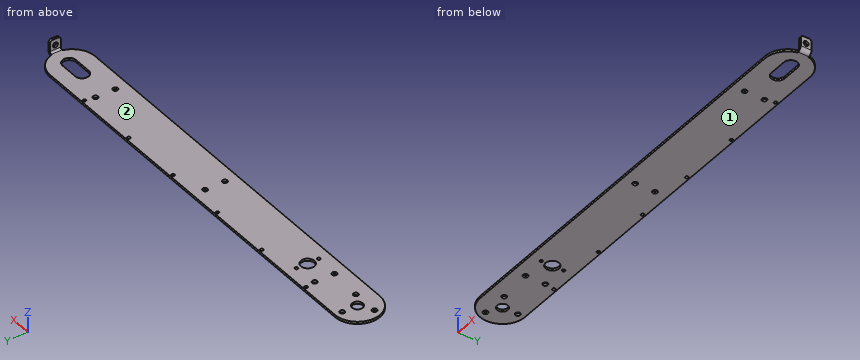
```python
from build123d import *
from build123d.topology import SkipClean

# Parameters (mm, degrees)
AUFSATZ_LINEAR_AUSTRAGEN1_DEPTH        = 2.5
SKIZZE7_W                              = 2.5
SKIZZE7_H                              = 6
AUFSATZ_LINEAR_AUSTRAGEN2_DEPTH        = 14
VERRUNDUNG2_R                          = 3
F_5_5_5_5_DURCHMESSER_BOHRUNG1_D       = 5.5
KREISMUSTER1_COUNT                     = 3
DURCHGANGSLOCH_F_R_M51_D               = 5.5
DURCHGANGSLOCH_F_R_M51_DEPTH           = 9.5
DURCHGANGSLOCH_F_R_M51_TIP             = 1.652366702
F_3_5_3_5_DURCHMESSER_BOHRUNG1_D       = 3.5
DURCHGANGSLOCH_F_R_M52_D               = 5.5
SPIEGELN2_AT_THE_SECOND_PLANE_COPY_1_D = 5.5
SCHNITT_LINEAR_AUSTRAGEN1_REACH        = 482.355
SKIZZE19_R                             = 7.5
VOLUMENK_RPER_START                    = -6
VOLUMENK_RPER_UMWANDELN1_DEPTH         = 12
VOLUMENK_RPER_UMWANDELN1_2_DEPTH       = 12


# Read off the part's stored shape, not the designer's step: Volumenkörper umwandeln1
with BuildPart() as part:
    # Skizze1 → Aufsatz-Linear austragen1 (new body)
    with BuildSketch(Plane.XY):
        with BuildLine():
            Line((-6, 0), (-25, 0))
            ThreePointArc((-25, 0), (-17.67766953, 17.67766953), (0, 25))
            Line((0, 25), (450, 25))
            ThreePointArc((450, 25), (465.411035007, 19.685019685), (474.269322199, 6))
            Line((474.269322199, 6), (479.5, 6))
            Line((479.5, 6), (479.5, 0))
            Line((479.5, 0), (477, 0))
            Line((477, 0), (475, 0))
            Line((475, 0), (462.5, 0))
            ThreePointArc((462.5, 0), (460.303300859, 5.303300859), (455, 7.5))
            Line((455, 7.5), (450, 7.5))
            Line((450, 7.5), (435, 7.5))
            ThreePointArc((435, 7.5), (429.696699141, 5.303300859), (427.5, 0))
            Line((427.5, 0), (6, 0))
            ThreePointArc((6, 0), (0, 6), (-6, 0))
        make_face()
    extrude(amount=-AUFSATZ_LINEAR_AUSTRAGEN1_DEPTH)

    # Skizze7 → Aufsatz-Linear austragen2 (add)
    with BuildSketch(Plane.XY):
        with Locations((478.25, 3)):
            Rectangle(SKIZZE7_W, SKIZZE7_H)
    extrude(amount=AUFSATZ_LINEAR_AUSTRAGEN2_DEPTH)

    # Verrundung2
    verrundung2_edges = [part.edges().sort_by_distance(p)[0] for p in [
        (478.25, 6, 14),
    ]]
    fillet(verrundung2_edges, radius=VERRUNDUNG2_R)

    # Spiegeln1: part across plane


with BuildPart() as part_1:
    with SkipClean():  # the faces are left unmerged after this step: merging them gives an invalid solid
        add(part.part)
        add(part.part.mirror(Plane(origin=(6, 0, -2.5), x_dir=(0, 0, 1), z_dir=(0, -1, 0))))

    # Ø5.5 (5.5) Durchmesser Bohrung1 (through all)
    with Locations(Plane.XY):
        with Locations((0, 17)):
            f_5_5_5_5_durchmesser_bohrung1 = Hole(F_5_5_5_5_DURCHMESSER_BOHRUNG1_D / 2)

    # Kreismuster1: Ø5.5 (5.5) Durchmesser Bohrung1 ×3 about axis
    with SkipClean():  # the faces are left unmerged after this step: merging them gives an invalid solid
        kreismuster1_axis = Axis((0, 0, 0), (0, 0, 1))
        for i in range(1, KREISMUSTER1_COUNT):
            add(f_5_5_5_5_durchmesser_bohrung1.rotate(kreismuster1_axis, i * 360 / KREISMUSTER1_COUNT), mode=Mode.SUBTRACT)

    # Durchgangsloch für M51
    with Locations(Plane(origin=(479.5, 0, 0), x_dir=(0, 0, -1), z_dir=(1, 0, 0))):
        with Locations((-7, 0)):
            Hole(DURCHGANGSLOCH_F_R_M51_D / 2, depth=DURCHGANGSLOCH_F_R_M51_DEPTH)
            with Locations((0, 0, -(DURCHGANGSLOCH_F_R_M51_DEPTH + DURCHGANGSLOCH_F_R_M51_TIP / 2))):  # 118° drill point
                Cone(0, DURCHGANGSLOCH_F_R_M51_D / 2, DURCHGANGSLOCH_F_R_M51_TIP, mode=Mode.SUBTRACT)

    # Ø3.5 (3.5) Durchmesser Bohrung1 (through all)
    with Locations(Plane.XY):
        with Locations((400, 22), (330, 22), (260, 22), (190, 22), (120, 22), (50, 22)):
            Hole(F_3_5_3_5_DURCHMESSER_BOHRUNG1_D / 2)

    # Durchgangsloch für M52 (through all)
    with Locations(Plane.XY):
        with Locations((52, 11), (225, 11)):
            durchgangsloch_f_r_m52 = Hole(DURCHGANGSLOCH_F_R_M52_D / 2)

    # Spiegeln2: Durchgangsloch für M52 across plane
    with SkipClean():  # the faces are left unmerged after this step: merging them gives an invalid solid
        add(durchgangsloch_f_r_m52.mirror(Plane(origin=(225, 0, 0), x_dir=(0, 0, 1), z_dir=(1, 0, 0))), mode=Mode.SUBTRACT)

    # Spiegeln2 at the second plane: Durchgangsloch für M52 across plane
    with SkipClean():  # the faces are left unmerged after this step: merging them gives an invalid solid
        add(durchgangsloch_f_r_m52.mirror(Plane.ZX), mode=Mode.SUBTRACT)

    # Spiegeln2 at the second plane copy 1 (through all)
    with Locations(Plane(origin=(450, 0, 0), x_dir=(-1, 0, 0), z_dir=(0, 0, 1))):
        with Locations((52, 11), (225, 11)):
            Hole(SPIEGELN2_AT_THE_SECOND_PLANE_COPY_1_D / 2)

    # Skizze19 → Schnitt-Linear austragen1 (cut, up to next)
    with BuildSketch(Plane.XY, mode=Mode.PRIVATE) as schnitt_linear_austragen1_sk1:
        with Locations((78.75, 0)):
            Circle(SKIZZE19_R)
    schnitt_linear_austragen1_tool1 = extrude(schnitt_linear_austragen1_sk1.sketch, amount=-SCHNITT_LINEAR_AUSTRAGEN1_REACH, mode=Mode.PRIVATE) & part_1.part
    add(schnitt_linear_austragen1_tool1.solids().sort_by_distance((78.75, 0, 0))[0], mode=Mode.SUBTRACT)

    # Skizze22 → Durchgangsloch für M31 (revolve, cut)
    with SkipClean():  # the faces are left unmerged after this step: merging them gives an invalid solid
        with BuildSketch(Plane(origin=(78.75, 12.5, 0), x_dir=(0, -1, 0), z_dir=(1, 0, 0))):
            Polygon((0, 0), (0, 3.771463052), (1.7, 2.75), (1.7, 0), align=None)
        durchgangsloch_f_r_m31 = revolve(axis=Axis((78.75, 12.5, 6.35), (0, 0, -1)), mode=Mode.SUBTRACT)

    # Spiegeln3: Durchgangsloch für M31 across plane
    with SkipClean():  # the faces are left unmerged after this step: merging them gives an invalid solid
        add(durchgangsloch_f_r_m31.mirror(Plane.ZX), mode=Mode.SUBTRACT)

    # Volumenkörper umwandeln1 outline → Volumenkörper umwandeln1 (cut)
    with SkipClean():  # the faces are left unmerged after this step: merging them gives an invalid solid
        with BuildSketch(Plane(origin=(0, 0, 0), x_dir=(1, 0, 0), z_dir=(0, 1, 0)).offset(VOLUMENK_RPER_START)):
            with BuildLine():
                Line((479.5, 2.5), (475, 2.5))
                ThreePointArc((475, 2.5), (478.181980515, 1.181980515), (479.5, -2))
                Line((479.5, -2), (479.5, 2.5))
            make_face()
        extrude(amount=VOLUMENK_RPER_UMWANDELN1_DEPTH, mode=Mode.SUBTRACT)

    # Volumenk_rper umwandeln1 2 outline → Volumenk_rper umwandeln1 2 (add)
    with BuildSketch(Plane(origin=(0, 0, 0), x_dir=(1, 0, 0), z_dir=(0, 1, 0)).offset(VOLUMENK_RPER_START)):
        with BuildLine():
            Line((477, 0), (475, 0))
            ThreePointArc((475, 0), (476.414213562, -0.585786438), (477, -2))
            Line((477, -2), (477, 0))
        make_face()
    extrude(amount=VOLUMENK_RPER_UMWANDELN1_2_DEPTH)


solid = part_1.part
```
The listing builds one solid part. Answer for the finished solid, in the listing's coordinates (mm). Face numbers are marked on the shaded views. A direction names the side the tool comes from. Coordinates: 2 decimals unless noted, no trailing zeros. Write each loop counter-clockwise with the first axis right and the second up, starting at its lowest first coordinate (ties: lowest second). Pieces come first, ordered by that corner, then holes.
Q1. Which of the six approach directions +Z, -Z, +X, -X, +Y, -Y give full straight-line access (tool end or side, diameter ignored) to the marked faces 1 and 2?
Returned:
face 1: -Z, +X, -X, +Y, -Y
face 2: +Z, -X, +Y, -Y
Q2. Find the intervals of material crossed by line 1 along Y through (x, z) = (78.75, -0.6); line 2 along Y through (x, z) = (477.55, 7); line 3 along Y through (x, z) = (120, -1.3), in increasing order.
Returned:
line 1: y = -25 to -14.2, -10.8 to -7.5, 7.5 to 10.8, 14.2 to 25
line 2: y = -6 to -2.75, 2.75 to 6
line 3: y = -25 to 20.25, 23.75 to 25
Q3. Given P1, Ø4.5, axis at x = 0, y = 17, coming from the +Z side; P2, Ø15, axis at x = 108.5, y = -7, coming from the +Z side; P3, Ø6.5, axis at y = 0, z = 7, coming from the -X side; P4, Ø1, axis at y = 0.5, z = 1, coming from the +X side, each flat-ended and moving along its own axis, determine where each tip first touches the part or whether it passes through.
Returned:
P1: passes through
P2: stops at z = 0
P3: stops at x = 477
P4: stops at x = 479.47
Q4. Section A-A, the plane x = 61 is taken. Write down the section's boundary in (y, z).
Returned:
outline: (-25, -2.5) - (25, -2.5) - (25, 0) - (-25, 0) - close
